CAD build for the part. Positions are in the model's coordinates, mm. Face numbers are marked on the shaded views. Round coordinates to 2 decimals unless told otherwise and drop trailing zeros. Loops run counter-clockwise (first coordinate to the right, second up) from the corner with the lowest first, then second, coordinate; pieces in that order, holes last. Notation, with made-up numbers: M 58.25,-20.75 L 78.25,-20.75 A11 ccw 78.25,-16.75 Z; hole C 80.25,58.5 d7. An arc over 180 degrees is marked long. Use one line per item in the form item = value.
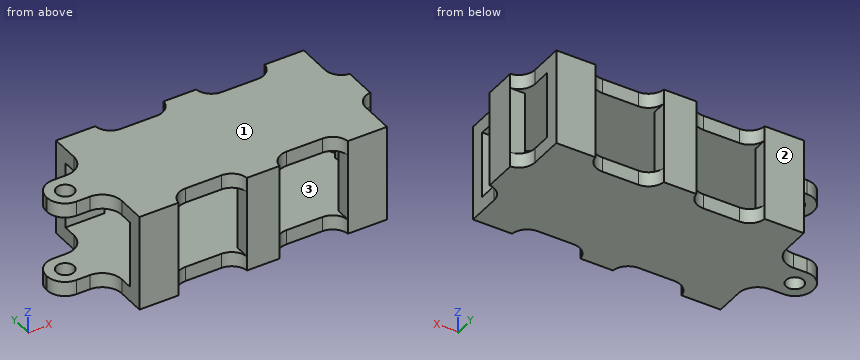
from build123d import *

# Parameters (mm, degrees)
F0_W        = 12
F0_H        = 4.5
F0_W_2      = 4.5
F0_H_2      = 5
F1_DEPTH    = 4.5
F2_DEPTH    = 20.5
F3_START    = 20.5
F3_DEPTH    = 4.5
F4_T1_DEPTH = 4.5
F4_T3_DEPTH = 4.5
F5_T1_DEPTH = 4.5
F5_T3_DEPTH = 4.5
F7_START    = -25
F6_W        = 15.7
F6_H        = 11.4
F6_R        = 2.7
F7_DEPTH    = 4.5
F8_DEPTH    = 4.5
F9_R        = 6
F10_R       = 5.5


# Not quite as in the source:
# - a fillet or chamfer that OpenCascade refuses, or shapes differently, is made with other operations: its cross-section is extruded or revolved along the edge and cut away or added


with BuildPart() as f1:
    # F0 (on Top) → F1 (new body)
    with BuildSketch(Plane.XY):
        Polygon((12, 31.6), (0, 31.6), (0, 0), (12, 0), (33, 0), (38, 0), (43, 0), (64, 0), (76, 0), (76, 10.8), (76, 15.8), (76, 20.8), (76, 31.6), (64, 31.6), (43, 31.6), (38, 31.6), (33, 31.6), align=None)
        with Locations((6, -2.25)):
            Rectangle(F0_W, F0_H)
        Polygon((38, 0), (33, 0), (33, -4.5), (43, -4.5), (43, 0), align=None)
        with Locations((70, -2.25)):
            Rectangle(F0_W, F0_H)
        with Locations((78.25, 13.3)):
            Rectangle(F0_W_2, F0_H_2)
        with Locations((78.25, 18.3)):
            Rectangle(F0_W_2, F0_H_2)
        with Locations((70, 33.85)):
            Rectangle(F0_W, F0_H)
        Polygon((33, 36.1), (33, 31.6), (38, 31.6), (43, 31.6), (43, 36.1), align=None)
        with Locations((6, 33.85)):
            Rectangle(F0_W, F0_H)
    extrude(amount=-F1_DEPTH)

    # F0 (on Top) → F2 (join)
    with BuildSketch(Plane.XY):
        with Locations((6, -2.25)):
            Rectangle(F0_W, F0_H)
        Polygon((38, 0), (33, 0), (33, -4.5), (43, -4.5), (43, 0), align=None)
        Polygon((33, 36.1), (33, 31.6), (38, 31.6), (43, 31.6), (43, 36.1), align=None)
        with Locations((6, 33.85)):
            Rectangle(F0_W, F0_H)
        with Locations((70, -2.25)):
            Rectangle(F0_W, F0_H)
        with Locations((78.25, 13.3)):
            Rectangle(F0_W_2, F0_H_2)
        with Locations((78.25, 18.3)):
            Rectangle(F0_W_2, F0_H_2)
        with Locations((70, 33.85)):
            Rectangle(F0_W, F0_H)
    extrude(amount=F2_DEPTH)

    # F0 (on Top) → F3 (join)
    with BuildSketch(Plane.XY.offset(F3_START)):
        with Locations((6, 33.85)):
            Rectangle(F0_W, F0_H)
        Polygon((12, 31.6), (0, 31.6), (0, 0), (12, 0), (33, 0), (38, 0), (43, 0), (64, 0), (76, 0), (76, 10.8), (76, 15.8), (76, 20.8), (76, 31.6), (64, 31.6), (43, 31.6), (38, 31.6), (33, 31.6), align=None)
        with Locations((6, -2.25)):
            Rectangle(F0_W, F0_H)
        Polygon((33, 36.1), (33, 31.6), (38, 31.6), (43, 31.6), (43, 36.1), align=None)
        Polygon((38, 0), (33, 0), (33, -4.5), (43, -4.5), (43, 0), align=None)
        with Locations((70, 33.85)):
            Rectangle(F0_W, F0_H)
        with Locations((70, -2.25)):
            Rectangle(F0_W, F0_H)
        with Locations((78.25, 18.3)):
            Rectangle(F0_W_2, F0_H_2)
        with Locations((78.25, 13.3)):
            Rectangle(F0_W_2, F0_H_2)
    extrude(amount=F3_DEPTH)

    # F4: fillet of radius 5 on 18 edges, made by hand

    # F4_s2 → F4_t1 (join)
    with BuildSketch(Plane.XY.offset(20.5)):
        with BuildLine():
            ThreePointArc((16.9749371855, 0), (13.6208352193, -1.2919007565), (12, -4.5))
            Line((12, -4.5), (12, 0))
            Line((12, 0), (16.9749371855, 0))
        make_face()
        with BuildLine():
            ThreePointArc((28.0250628145, 0), (31.3791647807, -1.2919007565), (33, -4.5))
            Line((33, -4.5), (33, 0))
            Line((33, 0), (28.0250628145, 0))
        make_face()
        with BuildLine():
            ThreePointArc((43, -4.5), (44.6208352193, -1.2919007565), (47.9749371855, 0))
            Line((47.9749371855, 0), (43, 0))
            Line((43, 0), (43, -4.5))
        make_face()
        with BuildLine():
            ThreePointArc((64, -4.5), (62.3791647807, -1.2919007565), (59.0250628145, 0))
            Line((59.0250628145, 0), (64, 0))
            Line((64, 0), (64, -4.5))
        make_face()
        with BuildLine():
            ThreePointArc((76, 5.8250628145), (77.2919007565, 9.1791647807), (80.5, 10.8))
            Line((80.5, 10.8), (76, 10.8))
            Line((76, 10.8), (76, 5.8250628145))
        make_face()
        with BuildLine():
            ThreePointArc((80.5, 20.8), (77.2919007565, 22.4208352193), (76, 25.7749371855))
            Line((76, 25.7749371855), (76, 20.8))
            Line((76, 20.8), (80.5, 20.8))
        make_face()
        with BuildLine():
            ThreePointArc((43, 36.1), (44.6208352193, 32.8919007565), (47.9749371855, 31.6))
            Line((47.9749371855, 31.6), (43, 31.6))
            Line((43, 31.6), (43, 36.1))
        make_face()
        with BuildLine():
            ThreePointArc((12, 36.1), (13.6208352193, 32.8919007565), (16.9749371855, 31.6))
            Line((16.9749371855, 31.6), (12, 31.6))
            Line((12, 31.6), (12, 36.1))
        make_face()
        with BuildLine():
            ThreePointArc((64, 36.1), (62.3791647807, 32.8919007565), (59.0250628145, 31.6))
            Line((59.0250628145, 31.6), (64, 31.6))
            Line((64, 31.6), (64, 36.1))
        make_face()
    extrude(amount=F4_T1_DEPTH)

    # F4_s4 → F4_t3 (join)
    with BuildSketch(Plane.XY.offset(-4.5)):
        with BuildLine():
            ThreePointArc((16.9749371855, 0), (13.6208352193, -1.2919007565), (12, -4.5))
            Line((12, -4.5), (12, 0))
            Line((12, 0), (16.9749371855, 0))
        make_face()
        with BuildLine():
            ThreePointArc((33, -4.5), (31.3791647807, -1.2919007565), (28.0250628145, 0))
            Line((28.0250628145, 0), (33, 0))
            Line((33, 0), (33, -4.5))
        make_face()
        with BuildLine():
            ThreePointArc((43, -4.5), (44.6208352193, -1.2919007565), (47.9749371855, 0))
            Line((47.9749371855, 0), (43, 0))
            Line((43, 0), (43, -4.5))
        make_face()
        with BuildLine():
            ThreePointArc((59.0250628145, 0), (62.3791647807, -1.2919007565), (64, -4.5))
            Line((64, -4.5), (64, 0))
            Line((64, 0), (59.0250628145, 0))
        make_face()
        with BuildLine():
            ThreePointArc((76, 5.8250628145), (77.2919007565, 9.1791647807), (80.5, 10.8))
            Line((80.5, 10.8), (76, 10.8))
            Line((76, 10.8), (76, 5.8250628145))
        make_face()
        with BuildLine():
            ThreePointArc((80.5, 20.8), (77.2919007565, 22.4208352193), (76, 25.7749371855))
            Line((76, 25.7749371855), (76, 20.8))
            Line((76, 20.8), (80.5, 20.8))
        make_face()
        with BuildLine():
            ThreePointArc((47.9749371855, 31.6), (44.6208352193, 32.8919007565), (43, 36.1))
            Line((43, 36.1), (43, 31.6))
            Line((43, 31.6), (47.9749371855, 31.6))
        make_face()
        with BuildLine():
            ThreePointArc((16.9749371855, 31.6), (13.6208352193, 32.8919007565), (12, 36.1))
            Line((12, 36.1), (12, 31.6))
            Line((12, 31.6), (16.9749371855, 31.6))
        make_face()
        with BuildLine():
            ThreePointArc((64, 36.1), (62.3791647807, 32.8919007565), (59.0250628145, 31.6))
            Line((59.0250628145, 31.6), (64, 31.6))
            Line((64, 31.6), (64, 36.1))
        make_face()
    extrude(amount=F4_T3_DEPTH)

    # F5: fillet of radius 5 on 2 edges, made by hand

    # F5_s2 → F5_t1 (join)
    with BuildSketch(Plane.XY.offset(20.5)):
        with BuildLine():
            ThreePointArc((33, 36.1), (31.3791647807, 32.8919007565), (28.0250628145, 31.6))
            Line((28.0250628145, 31.6), (33, 31.6))
            Line((33, 31.6), (33, 36.1))
        make_face()
    extrude(amount=F5_T1_DEPTH)

    # F5_s4 → F5_t3 (join)
    with BuildSketch(Plane.XY.offset(-4.5)):
        with BuildLine():
            ThreePointArc((33, 36.1), (31.3791647807, 32.8919007565), (28.0250628145, 31.6))
            Line((28.0250628145, 31.6), (33, 31.6))
            Line((33, 31.6), (33, 36.1))
        make_face()
    extrude(amount=F5_T3_DEPTH)

    # F6 (on face) → F7 (join)
    with BuildSketch(Plane.XY.offset(25).offset(F7_START)):
        with Locations((-7.85, 15.8)):
            Rectangle(F6_W, F6_H)
        with Locations((-10, 15.8)):
            Circle(F6_R, mode=Mode.SUBTRACT)
    extrude(amount=-F7_DEPTH)

    # F6 (on face) → F8 (join)
    with BuildSketch(Plane.XY.offset(25)):
        with Locations((-7.85, 15.8)):
            Rectangle(F6_W, F6_H)
        with Locations((-10, 15.8)):
            Circle(F6_R, mode=Mode.SUBTRACT)
    extrude(amount=-F8_DEPTH)

    # F9
    f9_edges = [f1.edges().sort_by_distance(p)[0] for p in [
        (0, 21.5, 22.75),
        (0, 10.1, 22.75),
        (0, 10.1, -2.25),
        (0, 21.5, -2.25),
    ]]
    fillet(f9_edges, radius=F9_R)

    # F10
    f10_edges = [f1.edges().sort_by_distance(p)[0] for p in [
        (-15.7, 21.5, 22.75),
        (-15.7, 10.1, 22.75),
        (-15.7, 10.1, -2.25),
        (-15.7, 21.5, -2.25),
    ]]
    fillet(f10_edges, radius=F10_R)


solid = f1.part
1. Pull direction Y, two halves, no side cores. Call the marked faces 1, 2 and 3: +Y half, -Y half, draft (parallel to the pull), parting line (faces both ways), or undercut.
Completed:
face_1 = draft
face_2 = +Y half
face_3 = undercut
2. Cut at B-B on z = 17.5. Write the cut outline in (x, y).
Completed:
outline = M 0,-4.5 L 12,-4.5 L 12,0 L 0,0 Z; M 0,31.6 L 12,31.6 L 12,36.1 L 0,36.1 Z; M 33,-4.5 L 43,-4.5 L 43,0 L 33,0 Z; M 33,31.6 L 43,31.6 L 43,36.1 L 33,36.1 Z; M 64,-4.5 L 76,-4.5 L 76,0 L 64,0 Z; M 64,31.6 L 76,31.6 L 76,36.1 L 64,36.1 Z; M 76,10.8 L 80.5,10.8 L 80.5,20.8 L 76,20.8 Z
3. Drop flat-ended pins along their axis: P1, Ø2, axis at x = 56, z = -3, coming from the -Y side; P2, Ø3, axis at y = 31, z = 14, coming from the -X side; P3, Ø8.5, axis at y = 3, z = 5, coming from the +X side. Give the stop position or say it passes through.
Completed:
P1 = 0
P2 = 0
P3 = 76
4. Cut at A-A on y = 29.5. Write the cut outline in (x, z).
Completed:
outline = M 0,-4.5 L 76,-4.5 L 76,0 L 0,0 Z; M 0,20.5 L 76,20.5 L 76,25 L 0,25 Z
5. Cut at C-C on x = 54. Write the cut outline in (y, z).
Completed:
outline = M 0,-4.5 L 31.6,-4.5 L 31.6,0 L 0,0 Z; M 0,20.5 L 31.6,20.5 L 31.6,25 L 0,25 Z
6. Probe line 1 along X through (y, z) = (-1.5, 6); line 2 along Y through (x, z) = (-10, 23.8); line 3 along Z through (x, y) = (14.5, -0.5). List the from-to ranges inside material, lowest first. Write a range as from..to.
Completed:
line_1 = 0..12, 33..43, 64..76
line_2 = 10.1..13.1, 18.5..21.5
line_3 = -4.5..0, 20.5..25
